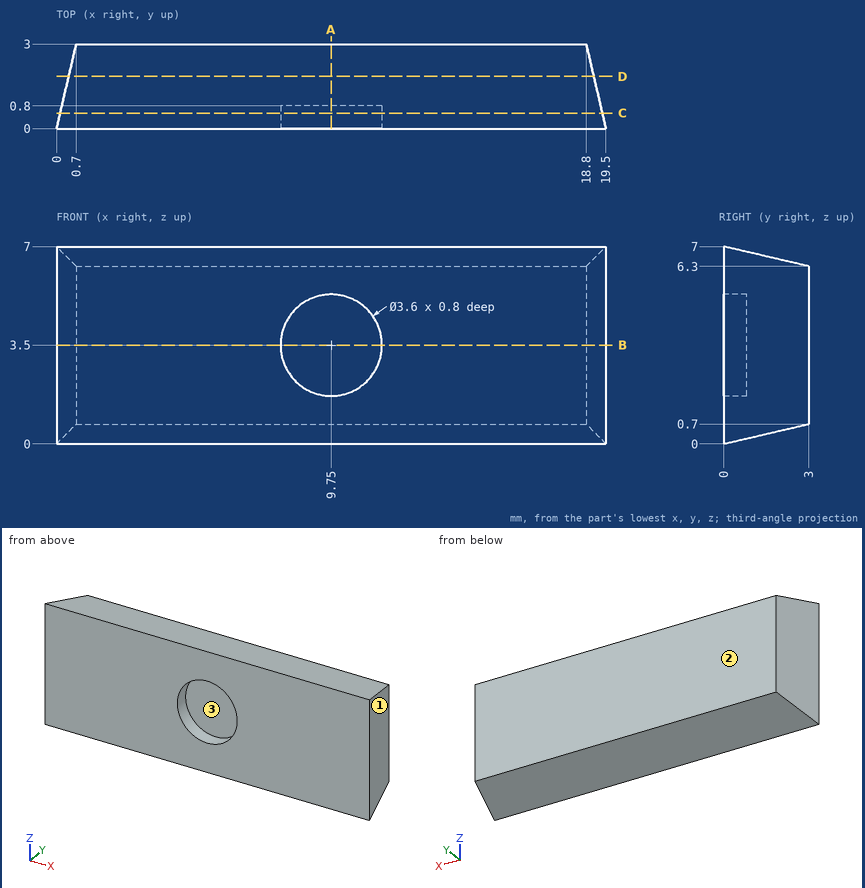
Geometry: see drawing. Coordinates: mm, zero at the bounding-box minimum. Give positions to 0.01 mm unless a question says otherwise; leave off trailing zeros. Order: outer loops, then holes, each group sorted by start corner. A loop starts at its lowest first (then second) coordinate and runs counter-clockwise, first axis right, second up. Notation, with made-up numbers: (38, 15) -> (60, 15) arc R25 ccw to (60, 42) -> close; hole circle Ø7 at (-1.5, 53). An arc over 180 degrees is marked (long way). Write each question's results on one line, items separated by ' | '.
1) Cut plane A-A (x = 9.75). Output: boundary loops of the cut face in (y, z), and give its area (3 significant figures).
Geometry says:
outline: (0, 0) -> (3, 0.7) -> (3, 6.3) -> (0, 7) -> (0, 5.3) -> (0.8, 5.3) -> (0.8, 1.7) -> (0, 1.7) -> close | area: 16.0 mm²
2) Cut plane D-D (y = 1.85). Output: boundary loops of the cut face in (x, z).
Geometry says:
outline: (0.43, 0.43) -> (19.07, 0.43) -> (19.07, 6.57) -> (0.43, 6.57) -> close
3) Line query: line 1 along X through (y, z) = (0.4, 3.5); line 2 along Y through (x, z) = (9.5, 3.25); line 3 along X through (y, z) = (0.5, 2.75). Output: solid intervals per line, ascending.
Geometry says:
line 1: x = 0.09 to 7.95, 11.55 to 19.41 | line 2: y = 0.8 to 3 | line 3: x = 0.12 to 8.11, 11.39 to 19.38
4) Cut plane B-B (z = 3.5). Output: boundary loops of the cut face in (x, y).
Geometry says:
outline: (0, 0) -> (7.95, 0) -> (7.95, 0.8) -> (11.55, 0.8) -> (11.55, 0) -> (19.5, 0) -> (18.8, 3) -> (0.7, 3) -> close
5) Cut plane C-C (y = 0.55). Output: boundary loops of the cut face in (x, z).
Geometry says:
outline: (0.13, 0.13) -> (19.37, 0.13) -> (19.37, 6.87) -> (0.13, 6.87) -> close; hole circle Ø3.6 at (9.75, 3.5)
6) First-contact query: pin 1 Ø3 at (x, z) = (9, 3.5) entering from -Y. Flat tip, straight axial feed; report the tip coordinate or a pass-through.
Geometry says:
pin 1: stops at y = 0
7) Draft query along X for the marked faces 1, 2 and 3. Return one class per face: released by +X, released by -X, zero draft, split by the parting line, or undercut.
Geometry says:
face 1: released by +X | face 2: zero draft | face 3: undercut
